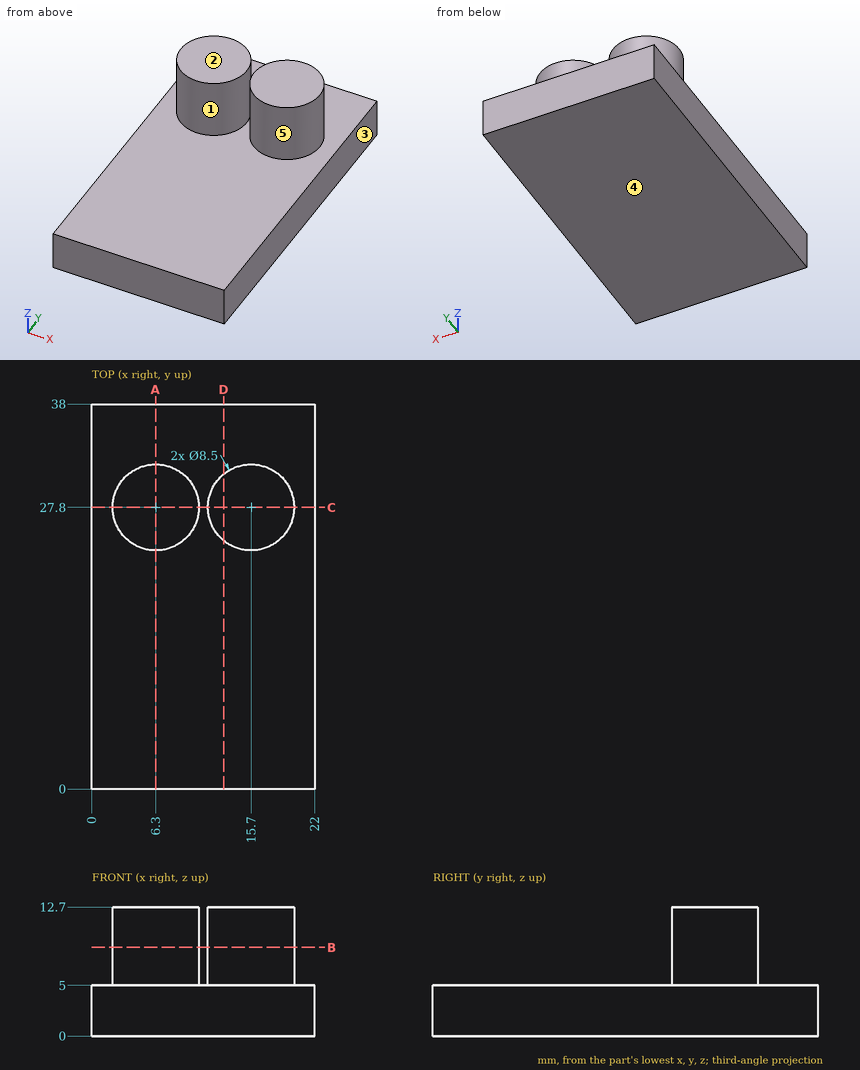
Study the drawing (mm; zero at the part's minimum x, y, z) and answer. A direction names the side the tool comes from. Round coordinates to 2 decimals unless told otherwise and drop trailing zeros. Loops run counter-clockwise (first coordinate to the right, second up) from the corner with the lowest first, then second, coordinate; pieces in that order, holes last.
Q1. Given pin 1 Ø5 at (y, z) = (17.5, 2) entering from -X; pin 2 Ø3 at (x, y) = (15, 19.5) entering from +Z, each flat-ended and moving along its own axis, determine where each tip first touches the part or whether it passes through.
Q2. Section B-B, the plane z = 8.75 is taken. Determine the outline of the cut face in (x, y), then the cut area to 3 significant figures.
Q3. Find the intervals of material crossed by line 1 (Z direction, x = 16.5, y = 20.5); line 2 (X direction, y = 29.5, z = 9.5); line 3 (Y direction, x = 5.25, z = 10), in increasing order.
Q4. Section C-C, the plane y = 27.8 is taken. Determine the outline of the cut face in (x, z).
Q5. Section D-D, the plane x = 13 is taken. Determine the outline of the cut face in (y, z), then the cut area to 3 significant figures.
Q6. Section A-A, the plane x = 6.3 is taken. Determine the outline of the cut face in (y, z), then the cut area to 3 significant figures.
Q7. For a pull along X with two mould halves and no side action, classify the marked faces 1, 2 and 3 as released by +X, released by -X, zero draft, split by the parting line, or undercut.
Q8. Which of the six approach directions +Z, -Z, +X, -X, +Y, -Y give full straight-line access (tool end or side, diameter ignored) to the marked faces 4 and 5?
Completed:
1. pin 1: stops at x = 0
1. pin 2: stops at z = 5
2. outline: circle Ø8.5 at (6.3, 27.8); circle Ø8.5 at (15.7, 27.8)
2. area: 113 mm2
3. line 1: z = 0 to 5
3. line 2: x = 2.4 to 10.2, 11.8 to 19.6
3. line 3: y = 23.68 to 31.92
4. outline: (0, 0) - (22, 0) - (22, 5) - (19.95, 5) - (19.95, 12.7) - (11.45, 12.7) - (11.45, 5) - (10.55, 5) - (10.55, 12.7) - (2.05, 12.7) - (2.05, 5) - (0, 5) - close
5. outline: (0, 0) - (38, 0) - (38, 5) - (31.08, 5) - (31.08, 12.7) - (24.52, 12.7) - (24.52, 5) - (0, 5) - close
5. area: 241 mm2
6. outline: (0, 0) - (38, 0) - (38, 5) - (32.05, 5) - (32.05, 12.7) - (23.55, 12.7) - (23.55, 5) - (0, 5) - close
6. area: 255 mm2
7. face 1: undercut
7. face 2: zero draft
7. face 3: released by +X
8. face 4: -Z, +X, -X, +Y, -Y
8. face 5: +Z
